Can you work these out from the model? Positions are in its coordinate system, mm. Face numbers are marked on the shaded views. A direction names the side the tool comes from. Round coordinates to 2 decimals unless told otherwise and drop trailing zeros. Order: outer loops, then holes, each group sorted by start corner. A loop starts at its lowest first (then second) coordinate and runs counter-clockwise, first axis right, second up. Notation, with made-up numbers: (-27, -10) - (27, -10) arc R27 ccw to (27, 17) - close; hole circle Ø9 at (47.5, -20). An arc over 180 degrees is marked (long way). Write item = value, one per line.
from build123d import *

# Parameters (mm, degrees)
F0_W        = 48.2
F0_H        = 48.2
F0_W_2      = 40.2
F0_H_2      = 40.2
F1_DEPTH    = 62
F3_START    = 20
F2_W        = 17
F2_H        = 50
F3_DEPTH    = 5
F4_T        = 2.5
F4_T3_DEPTH = 49.1321159601
F4_T5_DEPTH = 22
F4_T7_DEPTH = 9
F4_T9_DEPTH = 67


# Not quite as in the source:
# - a shell that OpenCascade refuses in one call is made with other operations: the cavity is built on its own and cut out


with BuildPart() as f1:
    # F0 (on Front) → F1 (new body)
    with BuildSketch(Plane.XZ):
        Rectangle(F0_W, F0_H)
        Rectangle(F0_W_2, F0_H_2, mode=Mode.SUBTRACT)
    extrude(amount=F1_DEPTH)

    # F2 (on Top) → F3 (join)
    with BuildSketch(Plane.XY.offset(F3_START)):
        with Locations((0, -42.8678840399)):
            Rectangle(F2_W, F2_H)
    extrude(amount=F3_DEPTH)

    # F4: shell of thickness 2.5, made by hand


with BuildPart() as f4_core1:
    # F4_t2: copy of F1
    add(f1.part)

    # the walls: a layer under each face that stays
    f4_faces = [f4_core1.faces().sort_by_distance(p)[0] for p in [
        (24.1, -31, 0),
        (0, -31, -24.1),
        (16.0666666667, -51.6666666667, 24.1),
        (-20.6571428571, 0, -20.6571428571),
        (-20.6571428571, -62, -20.6571428571),
        (-24.1, -31, 0),
        (-8.5, -26.2012173732, 24.1666666667),
        (0, -17.8678840399, 24.55),
        (8.5, -59.5345507065, 24.1666666667),
        (20.1, -31, 0),
        (0, -31, -20.1),
        (-20.1, -31, 0),
        (-13.4, -51.6666666667, 20.1),
        (0, -67.8678840399, 22.5),
        (0, -17.8678840399, 20.05),
    ]]
    thicken(f4_faces, amount=-F4_T, mode=Mode.SUBTRACT)

    # F4_s4 → F4_t3 (cut)
    with BuildSketch(Plane.XZ.offset(15.3678840399)):
        Polygon((-8.525, 24.125), (-8.5, 21.6), (-6, 21.6), (-6, 24.1), align=None)
        Polygon((8.525, 24.125), (8.5, 21.6), (6, 21.6), (6, 24.1), align=None)
        Polygon((-8.525, 20.075), (-6, 20.1), (-6, 22.6), (-8.5, 22.6), align=None)
        Polygon((8.525, 20.075), (6, 20.1), (6, 22.6), (8.5, 22.6), align=None)
    extrude(amount=F4_T3_DEPTH, mode=Mode.SUBTRACT)

    # F4_s6 → F4_t5 (cut)
    with BuildSketch(Plane.YZ.offset(-11)):
        Polygon((-17.8428840399, 24.125), (-17.8678840399, 21.6), (-20.3678840399, 21.6), (-20.3678840399, 24.1), align=None)
        Polygon((-17.8428840399, 20.075), (-17.8678840399, 22.6), (-20.3678840399, 22.6), (-20.3678840399, 20.1), align=None)
    extrude(amount=F4_T5_DEPTH, mode=Mode.SUBTRACT)

    # F4_s8 → F4_t7 (cut)
    with BuildSketch(Plane.XY.offset(17.6)):
        Polygon((-8.525, -62.025), (-8.5, -59.5), (-6, -59.5), (-6, -62), align=None)
        Polygon((8.525, -62.025), (8.5, -59.5), (6, -59.5), (6, -62), align=None)
    extrude(amount=F4_T7_DEPTH, mode=Mode.SUBTRACT)

    # F4_s10 → F4_t9 (cut)
    with BuildSketch(Plane.XZ.offset(-2.5)):
        Polygon((20.075, 20.075), (22.6, 20.1), (22.6, 22.6), (20.1, 22.6), align=None)
        Polygon((20.075, -20.075), (22.6, -20.1), (22.6, -22.6), (20.1, -22.6), align=None)
        Polygon((-20.075, -20.075), (-20.1, -22.6), (-22.6, -22.6), (-22.6, -20.1), align=None)
        Polygon((-20.075, 20.075), (-22.6, 20.1), (-22.6, 22.6), (-20.1, 22.6), align=None)
    extrude(amount=F4_T9_DEPTH, mode=Mode.SUBTRACT)


with BuildPart() as f1_1:
    add(f1.part)

    # what is left inside the walls is the cavity
    f4_cavity = [f4_core1.part.solids().sort_by_distance(p)[0] for p in [
        (0, -50.367884, 20.025),
    ]]
    add(f4_cavity, mode=Mode.SUBTRACT)


solid = f1_1.part
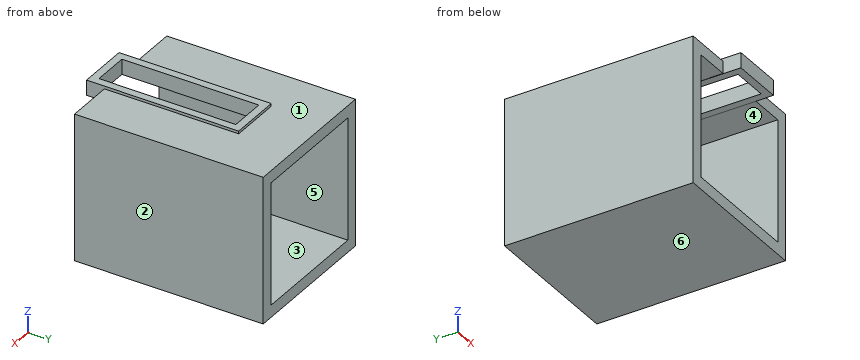
(1) Thinking about a two-plate mould opening in X: for the marked faces 1, 2 and 3, which applies, +X half, -X half, draft (parallel to the pull), parting line (faces both ways), or undercut?
Computed:
face_1 = draft
face_2 = +X half
face_3 = undercut
(2) If we section it at A-A (x = -3.5): Write out the boundary of the cut face in (y, z), plus the area to 3 significant figures.
Computed:
outline = (-67.87, 20) - (-65.37, 20) - (-65.37, 25) - (-67.87, 25) - close; (-62, -24.1) - (0, -24.1) - (0, -20.1) - (-62, -20.1) - close; (-20.37, 20) - (-17.87, 20) - (-17.87, 20.1) - (0, 20.1) - (0, 24.1) - (-17.87, 24.1) - (-17.87, 25) - (-20.37, 25) - close
area = 344 mm^2
(3) If we section it at B-B (z = 19): Write out the boundary of the cut face in (x, y), plus the area to 3 significant figures.
Computed:
outline = (-24.1, -62) - (-20.1, -62) - (-20.1, 0) - (-24.1, 0) - close; (20.1, -62) - (24.1, -62) - (24.1, 0) - (20.1, 0) - close
area = 496 mm^2
(4) Will these pins go through, and if not, where does the flat tip stop? P1, Ø6, axis at x = 15, y = -15.5, coming from the +Z side; P2, Ø5, axis at x = 18, z = 11, coming from the -Y side.
Computed:
P1 = 24.1
P2 = -62
(5) If we section it at D-D (x = 11): Write out the boundary of the cut face in (y, z).
Computed:
outline = (-62, -24.1) - (0, -24.1) - (0, -20.1) - (-62, -20.1) - close; (-62, 20.1) - (0, 20.1) - (0, 24.1) - (-62, 24.1) - close
(6) If I drill on line 1 (Z direction, x = -12.5, y = -60); line 2 (Z direction, x = -8, y = -35), over which ranges is the centre line in solid material (lowest first)? Write a range as from..to.
Computed:
line_1 = -24.1..-20.1, 20.1..24.1
line_2 = -24.1..-20.1, 20..25
(7) On a 3-axis mill with a long thin cutter (end or side, diameter ignored), from which of +Z, -Z, +X, -X, +Y, -Y can I reach the whole of each face in a straight line? I mean the marked faces 4, 5 and 6. Say none if no direction works.
Computed:
face_4 = +Y
face_5 = +Y, -Y
face_6 = -Z, +X, -X, +Y, -Y
(8) If we section it at C-C (y = -15): Write out the boundary of the cut face in (x, z).
Computed:
outline = (-24.1, -24.1) - (24.1, -24.1) - (24.1, 24.1) - (-24.1, 24.1) - close; hole (-20.1, -20.1) - (20.1, -20.1) - (20.1, 20.1) - (-20.1, 20.1) - close
